CAD build for the part. Positions are in the model's coordinates, mm. A direction names the side the tool comes from. Coordinates: 2 decimals unless noted, no trailing zeros. Loops run counter-clockwise (first coordinate to the right, second up) from the corner with the lowest first, then second, coordinate; pieces in that order, holes last. Notation, with made-up numbers: (-20, 72.5) -> (27, 72.5) arc R20 cw to (27, 86.5) -> close; hole circle Ø11 at (72, 0.5). An arc over 180 degrees is marked (long way). Write each question's results on one line, items separated by ' | '.
```python
from build123d import *

# Parameters (mm, degrees)
SKETCH1_R               = 3
BOSS_EXTRUDE1_DEPTH     = 45
SKETCH2_R               = 5
BOSS_EXTRUDE2_DEPTH     = 2
CUT_EXTRUDE1_DEPTH      = 48.528938553
CUT_EXTRUDE1_DEPTH_BACK = 48.528938553
SKETCH3_R               = 1
SKETCH4_R               = 1.5
CUT_EXTRUDE2_DEPTH      = 45


with BuildPart() as part:
    # Sketch1 → Boss-Extrude1 (new body)
    with BuildSketch(Plane.XY):
        with Locations(Location((0, 0, 0), (0, 0, 180))):
            Circle(SKETCH1_R)
    extrude(amount=BOSS_EXTRUDE1_DEPTH)

    # Sketch2 → Boss-Extrude2 (add)
    with BuildSketch(Plane.XY.offset(45)):
        Circle(SKETCH2_R)
    extrude(amount=BOSS_EXTRUDE2_DEPTH)

    # Sketch3 → Cut-Extrude1 (cut, two sides: drawn at the far end of the back side and taken through both)
    with BuildSketch(Plane(origin=(0, 0, 0), x_dir=(1, 0, 0), z_dir=(0, 1, 0)).offset(-CUT_EXTRUDE1_DEPTH_BACK)):
        with Locations(Location((0, -3.5, 0), (0, 0, 270))):
            Circle(SKETCH3_R)
    extrude(amount=CUT_EXTRUDE1_DEPTH + CUT_EXTRUDE1_DEPTH_BACK, mode=Mode.SUBTRACT)

    # Sketch4 → Cut-Extrude2 (cut)
    with BuildSketch(Plane(origin=(0, 0, 0), x_dir=(-1, 0, 0), z_dir=(0, 0, -1))):
        Circle(SKETCH4_R)
    extrude(amount=-CUT_EXTRUDE2_DEPTH, mode=Mode.SUBTRACT)


solid = part.part
```
Q1. Cut at B-B on y = 0. Write the cut outline in (x, z), and give its area (3 significant figures).
Results are:
outline: (-5, 45) -> (-3, 45) -> (-3, 0) -> (-1.5, 0) -> (-1.5, 45) -> (1.5, 45) -> (1.5, 0) -> (3, 0) -> (3, 45) -> (5, 45) -> (5, 47) -> (-5, 47) -> close | area: 155 mm^2
Q2. Wall check: L1, parallel to Y at x = 0, z = 20; L2, parallel to Z at x = 0, y = -2.5; L3, parallel to Z at x = -1, y = 3.75. Give the ranges that are in metal, low to high. Write a range as from..to.
Results are:
L1: -3..-1.5, 1.5..3 | L2: 0..2.5, 4.5..47 | L3: 45..47
Q3. Which spindle directions (+Z, -Z, +X, -X, +Y, -Y) get a long thin tool onto all of the face, cutting with end or side? Do faces 1 (the cylindrical face through (0, 2, 2.5)), 2 (the cylindrical face through (-2.86, -0.9, 22.18)). Say none if no direction does.
Results are:
face 1: +Y, -Y | face 2: -Z
Q4. Drop flat-ended pins along their axis: pin 1 (5 mm diameter, centred on x = -0.5, z = 41, fed in from -Y); pin 2 (6 mm diameter, centred on x = 1.5, y = 3, fed in from -Z); pin 3 (1.5 mm diameter, centred on x = 0.5, y = 0, fed in from -Z); pin 4 (2 mm diameter, centred on y = -3.5, z = 32.5, fed in from +X). Give the stop position or say it passes through.
Results are:
pin 1: y = -3 | pin 2: z = 0 | pin 3: z = 45 | pin 4: x = 1.66
Q5. Cut at D-D on y = 2.5. Write the cut outline in (x, z), and give its area (3 significant figures).
Results are:
outline: (-4.33, 45) -> (-1.66, 45) -> (-1.66, 0) -> (1.66, 0) -> (1.66, 45) -> (4.33, 45) -> (4.33, 47) -> (-4.33, 47) -> close; hole circle Ø2 at (0, 3.5) | area: 163 mm^2
Q6. Cut at A-A on x = 0. Write the cut outline in (y, z), and give its area (3 significant figures).
Results are:
outline: (-5, 45) -> (-3, 45) -> (-3, 4.5) -> (-1.5, 4.5) -> (-1.5, 45) -> (1.5, 45) -> (1.5, 4.5) -> (3, 4.5) -> (3, 45) -> (5, 45) -> (5, 47) -> (-5, 47) -> close; (-3, 0) -> (-1.5, 0) -> (-1.5, 2.5) -> (-3, 2.5) -> close; (1.5, 0) -> (3, 0) -> (3, 2.5) -> (1.5, 2.5) -> close | area: 149 mm^2
Q7. Cut at C-C on z = 3.5. Write the cut outline in (x, y), and give its area (3 significant figures).
Results are:
outline: (-1, -2.83) -> (-1, -1.12) arc R1.5 cw to (-1, 1.12) -> (-1, 2.83) arc R3 ccw to start; (1, -2.83) arc R3 ccw to (1, 2.83) -> (1, 1.12) arc R1.5 cw to (1, -1.12) -> close | area: 15.0 mm^2
Q8. Pull direction Z, two halves, no side cores. Call faces 3 (the cylindrical face through (1.5, 0.07, 22.18)), 4 (the flat face through (-0.1, -3.3, 45)), 5 (the cylindrical face through (-0.6, -2.1, 2.7)): +Z half, -Z half, draft (parallel to the pull), parting line (faces both ways), or undercut.
Results are:
face 3: draft | face 4: -Z half | face 5: undercut
